CAD build for the part. Positions are in the model's coordinates, mm. A direction names the side the tool comes from. Coordinates: 2 decimals unless noted, no trailing zeros. Order: outer loops, then holes, each group sorted by start corner. A loop starts at its lowest first (then second) coordinate and runs counter-clockwise, first axis right, second up. Notation, with made-up numbers: M 71,-38 L 84,-38 A20 cw 84,-33 Z; hole C 28,-0.75 d7. An arc over 180 degrees is marked long. One line per item, written item: value.
from build123d import *

# Parameters (mm, degrees)
BOSS_EXTRUDE1_DEPTH = 9
SKETCH5_W           = 5
SKETCH5_H           = 30
SKETCH5_W_2         = 15
SKETCH5_H_2         = 5
CUT_EXTRUDE2_DEPTH  = 9


with BuildPart() as part:
    # Sketch2 → Boss-Extrude1 (new body)
    with BuildSketch(Plane.XY):
        Polygon((-151.004642906, 60), (-160.004642906, 60), (-160.004642906, 0), (-151.004642906, 0), (-151.004642906, -60), (-160.004642906, -60), (-160.004642906, -120), (-151.004642906, -120), (-151.004642906, -190), (-81.004642906, -190), (-81.004642906, -199), (-21.004642906, -199), (-21.004642906, -190), (38.995357094, -190), (38.995357094, -199), (98.995357094, -199), (98.995357094, -190), (168.995357094, -190), (168.995357094, -120), (177.995357094, -120), (177.995357094, -60), (168.995357094, -60), (168.995357094, 0), (177.995357094, 0), (177.995357094, 60), (168.995357094, 60), (168.995357094, 130), (168.995357094, 139), (98.995357094, 139), (38.995357094, 139), (38.995357094, 130), (-21.004642906, 130), (-21.004642906, 139), (-81.004642906, 139), (-81.004642906, 130), (-151.004642906, 130), align=None)
    extrude(amount=BOSS_EXTRUDE1_DEPTH)

    # Sketch5 → Cut-Extrude2 (cut)
    with BuildSketch(Plane.XY.offset(9)):
        with Locations((92.864342421, -142)):
            Rectangle(SKETCH5_W, SKETCH5_H)
        with Locations((-59.699642906, -10.5)):
            Rectangle(SKETCH5_W_2, SKETCH5_H_2)
        with Locations((-74.873628233, -62)):
            Rectangle(SKETCH5_W, SKETCH5_H)
        with Locations((-74.873628233, -142)):
            Rectangle(SKETCH5_W, SKETCH5_H)
        with Locations((92.864342421, -62)):
            Rectangle(SKETCH5_W, SKETCH5_H)
        with Locations((77.690357094, -10.5)):
            Rectangle(SKETCH5_W_2, SKETCH5_H_2)
    extrude(amount=-CUT_EXTRUDE2_DEPTH, mode=Mode.SUBTRACT)


solid = part.part
Q1. Which spindle directions (+Z, -Z, +X, -X, +Y, -Y) get a long thin tool onto all of the face, cutting with end or side? Do faces 1 (the face through (-151.005, -30, 4)), 2 (the face through (-116, -190, 4)), 3 (the face through (9, 130, 4)). Say none if no direction does.
Recorded:
face 1: +Z, -Z, -X
face 2: +Z, -Z, -X, -Y
face 3: +Z, -Z, +Y
Q2. Drill centre lines: line 1 along X through (y, z) = (-140, 3.25); line 2 along X through (y, z) = (-9, 2.5); line 3 along Y through (x, z) = (-123.5, 8.75). Where is each one in solid material? Low to high.
Recorded:
line 1: x = -151 to -77.37, -72.37 to 90.36, 95.36 to 169
line 2: x = -151 to -67.2, -52.2 to 70.19, 85.19 to 169
line 3: y = -190 to 130
Q3. Slice it at C-C (z = 2.75). Give the number of separate pieces and of enclosed holes in the cut face, plus the area to 3 significant figures.
Recorded:
separate pieces: 1
enclosed holes: 6
area: 107,000 mm^2
Q4. Pin check, flat tips, straight feed: pin 1 Ø2 at (x, z) = (116.5, 7.5) entering from -Y; pin 2 Ø4.5 at (y, z) = (-170.5, 5.5) entering from -X; pin 3 Ø2 at (x, z) = (15, 7) entering from +Y. Stop position of each tip, or through.
Recorded:
pin 1: stops at y = -190
pin 2: stops at x = -151
pin 3: stops at y = 130
Q5. Slice it at B-B (x = 15.5). List the corners of the cut face in (y, z), plus the area to 3 significant figures.
Recorded:
outline: M -190,0 L 130,0 L 130,9 L -190,9 Z
area: 2,880 mm^2
Q6. Slice it at A-A (y = -148.5). List the corners of the cut face in (x, z), plus the area to 3 significant figures.
Recorded:
outline: M -151,0 L -77.37,0 L -77.37,9 L -151,9 Z; M -72.37,0 L 90.36,0 L 90.36,9 L -72.37,9 Z; M 95.36,0 L 169,0 L 169,9 L 95.36,9 Z
area: 2,790 mm^2
Q7. Mould opens along X. For faces 4 (the face through (-155, -60, 4)), 5 (the face through (168.995, -30, 4)), 6 (the face through (95.364, -142, 5)) say: released by +X, released by -X, zero draft, split by the parting line, or undercut.
Recorded:
face 4: zero draft
face 5: released by +X
face 6: undercut
Q8. Slice it at D-D (y = 88). List the corners of the cut face in (x, z).
Recorded:
outline: M -151,0 L 169,0 L 169,9 L -151,9 Z
